Work out the finished part from the listing and answer in its coordinate system (mm). A direction names the side the tool comes from. Coordinates: 2 decimals unless noted, no trailing zeros. Write each loop counter-clockwise with the first axis right and the second up, starting at its lowest first coordinate (ties: lowest second). Pieces come first, ordered by that corner, then holes. Notation, with made-up numbers: (13, 56.5) - (52, 56.5) arc R9 ccw to (52, 60.5) - close; hole circle Ø9 at (21, -8). An arc over 180 degrees is marked (long way). Use one line per item in the form item = value. Start each with the question number.
Item 1: For faces 1 (the flat face through (-60.7, 0, 3)), 2 (the flat face through (60.2, 0, 10)), 3 (the flat face through (62.2, 0, 6)), determine the directions among +Z, -Z, +X, -X, +Y, -Y from which every point of the face is accessible in a straight line to the end or side of a thin tool.
Item 2: A cutting plane is placed at D-D (z = 4). Write down the section's boundary in (x, y), then the cut area to 3 significant figures.
Item 3: A cutting plane is placed at C-C (x = -32.5). Write down the section's boundary in (y, z).
Item 4: Determine the mould class of faces 4 (the flat face through (-62.2, 0, 6)), 5 (the flat face through (-1, -23.7, 6)), 6 (the flat face through (-1, 22.2, 3)) for opening direction X: released by +X, released by -X, zero draft, split by the parting line, or undercut.
Item 5: Consider probe 1 along X at (y, z) = (2.5, 1.25); probe 2 along Y at (x, z) = (44, 5.75); probe 3 along X at (y, z) = (-15, 10). Determine where each line is inside the solid, lowest interval first.
Item 6: A cutting plane is placed at A-A (y = 13.5). Write down the section's boundary in (x, z).
Item 7: A cutting plane is placed at B-B (z = 11). Write down the section's boundary in (x, y).
from build123d import *

# Parameters (mm, degrees)
F0_W     = 124.4
F0_H     = 47.4
F0_W_2   = 121.4
F0_H_2   = 44.4
F1_DEPTH = 7
F2_W     = 124.4
F2_H     = 47.4
F2_W_2   = 121.4
F2_H_2   = 44.4
F2_W_3   = 120.4
F2_H_3   = 40.4
F3_DEPTH = 6


with BuildPart() as f1:
    # F0 (on Top) → F1 (new body)
    with BuildSketch(Plane.XY):
        Rectangle(F0_W, F0_H)
        Rectangle(F0_W_2, F0_H_2, mode=Mode.SUBTRACT)
    extrude(amount=F1_DEPTH)

    # F2 (on face) → F3 (join)
    with BuildSketch(Plane.XY.offset(7)):
        Rectangle(F2_W, F2_H)
        Rectangle(F2_W_2, F2_H_2, mode=Mode.SUBTRACT)
        Rectangle(F2_W_2, F2_H_2)
        Rectangle(F2_W_3, F2_H_3, mode=Mode.SUBTRACT)
    extrude(amount=F3_DEPTH)


solid = f1.part
Answer:
q1.face_1 = -Z
q1.face_2 = +Z, -Z
q1.face_3 = +Z, -Z, +X, +Y, -Y
q2.outline = (-62.2, -23.7) - (62.2, -23.7) - (62.2, 23.7) - (-62.2, 23.7) - close; hole (-60.7, -22.2) - (60.7, -22.2) - (60.7, 22.2) - (-60.7, 22.2) - close
q2.area = 506 mm²
q3.outline = (-23.7, 0) - (-22.2, 0) - (-22.2, 7) - (-20.2, 7) - (-20.2, 13) - (-23.7, 13) - close; (20.2, 7) - (22.2, 7) - (22.2, 0) - (23.7, 0) - (23.7, 13) - (20.2, 13) - close
q4.face_4 = released by -X
q4.face_5 = zero draft
q4.face_6 = undercut
q5.probe_1 = -62.2 to -60.7, 60.7 to 62.2
q5.probe_2 = -23.7 to -22.2, 22.2 to 23.7
q5.probe_3 = -62.2 to -60.2, 60.2 to 62.2
q6.outline = (-62.2, 0) - (-60.7, 0) - (-60.7, 7) - (-60.2, 7) - (-60.2, 13) - (-62.2, 13) - close; (60.2, 7) - (60.7, 7) - (60.7, 0) - (62.2, 0) - (62.2, 13) - (60.2, 13) - close
q7.outline = (-62.2, -23.7) - (62.2, -23.7) - (62.2, 23.7) - (-62.2, 23.7) - close; hole (-60.2, -20.2) - (60.2, -20.2) - (60.2, 20.2) - (-60.2, 20.2) - close
